from build123d import *

# Parameters (mm, degrees)
BOSS_EXTRUDE1_DEPTH = 3.175


with BuildPart() as part:
    # Sketch1 → Boss-Extrude1 (new body)
    with BuildSketch(Plane.XY):
        with BuildLine():
            Line((0, 0), (0, 3.175))
            Line((0, 3.175), (-3.175, 3.175))
            Line((-3.175, 3.175), (-3.175, 6.35))
            Line((-3.175, 6.35), (0, 6.35))
            Line((0, 6.35), (0, 7.62))
            Line((0, 7.62), (9.525, 7.62))
            Line((9.525, 7.62), (9.525, 5.582477749))
            Line((9.525, 5.582477749), (12.7, 5.582477749))
            Line((12.7, 5.582477749), (12.7, 7.62))
            Line((12.7, 7.62), (14.224, 7.62))
            Line((14.224, 7.62), (14.224, 11.43))
            Line((14.224, 11.43), (12.7, 11.43))
            Line((12.7, 11.43), (12.7, 13.467522251))
            Line((12.7, 13.467522251), (9.525, 13.467522251))
            Line((9.525, 13.467522251), (9.525, 11.43))
            Line((9.525, 11.43), (0, 11.43))
            Line((0, 11.43), (0, 12.7))
            Line((0, 12.7), (-3.175, 12.7))
            Line((-3.175, 12.7), (-3.175, 15.875))
            Line((-3.175, 15.875), (0, 15.875))
            Line((0, 15.875), (0, 19.05))
            Line((0, 19.05), (3.175, 19.05))
            Line((3.175, 19.05), (3.175, 22.225))
            Line((3.175, 22.225), (12.7, 22.225))
            Line((12.7, 22.225), (12.7, 19.05))
            Line((12.7, 19.05), (15.875, 19.05))
            ThreePointArc((15.875, 19.05), (29.345384182, 13.470384182), (34.925, 0))
            Line((34.925, 0), (25.4, 0))
            Line((25.4, 0), (25.4, -3.175))
            Line((25.4, -3.175), (15.875, -3.175))
            Line((15.875, -3.175), (15.875, 0))
            Line((15.875, 0), (0, 0))
        make_face()
    extrude(amount=BOSS_EXTRUDE1_DEPTH)


solid = part.part
For this review, take the finished solid that the model builds, in its own axes (mm). A direction names the side the tool comes from. Give positions to 0.01 mm unless a question says otherwise; leave off trailing zeros. Loops run counter-clockwise (first coordinate to the right, second up) from the corner with the lowest first, then second, coordinate; pieces in that order, holes last. Notation, with made-up numbers: (75.25, 84) - (131.25, 84) arc R16 cw to (131.25, 113) - close; hole circle Ø3 at (71.25, 63.5). An arc over 180 degrees is marked (long way). Write each question's results on one line, items separated by ' | '.
(1) Take a section at C-C (y = -1). Give the boundary of the cut face in (x, z) (3 decimals), then the cut area to 3 significant figures.
Conclusion:
outline: (15.875, 0) - (25.4, 0) - (25.4, 3.175) - (15.875, 3.175) - close | area: 30.2 mm^2
(2) Take a section at A-A (x = 2.5). Give the boundary of the cut face in (y, z) (3 decimals), then the cut area to 3 significant figures.
Conclusion:
outline: (0, 0) - (7.62, 0) - (7.62, 3.175) - (0, 3.175) - close; (11.43, 0) - (19.05, 0) - (19.05, 3.175) - (11.43, 3.175) - close | area: 48.4 mm^2
(3) For pin 1 Ø1.2 at (x, z) = (13.5, 2.5) entering from -Y; pin 2 Ø1.6 at (x, z) = (-1, 1) entering from -Y (3 decimals); pin 3 Ø1 at (y, z) = (-1, 2) entering from -X (3 decimals); pin 4 Ø0.6 at (y, z) = (12.5, 1.5) entering from -X (3 decimals), all flat-tipped, find the tip position at first contact; note any pin that passes through.
Conclusion:
pin 1: y = 0 | pin 2: y = 3.175 | pin 3: x = 15.875 | pin 4: x = -3.175
(4) Draft analysis for pull direction Y (two halves, no side actions). For faces 1 (the flat face through (-2, 15.875, 2)), 2 (the flat face through (15.875, -2, 2)), 3 (the flat face through (9.525, 7, 2)), state which applies: +Y half, -Y half, draft (parallel to the pull), parting line (faces both ways), or undercut.
Conclusion:
face 1: +Y half | face 2: draft | face 3: undercut
(5) For line 1 along Y through (x, z) = (12, 1) (3 decimals); line 2 along Y through (x, z) = (-1, 1.6) (3 decimals); line 3 along X through (y, z) = (19.5, 0.5) (3 decimals), list the stretches that pass through material, from the lowest coordinate up.
Conclusion:
line 1: 0 to 5.582, 13.468 to 22.225 | line 2: 3.175 to 6.35, 12.7 to 15.875 | line 3: 3.175 to 12.7
(6) Take a section at D-D (x = 22). Give the boundary of the cut face in (y, z) (3 decimals), then the cut area to 3 significant figures.
Conclusion:
outline: (-3.175, 0) - (18.038, 0) - (18.038, 3.175) - (-3.175, 3.175) - close | area: 67.4 mm^2
(7) For faces 4 (the flat face through (0, 17, 2)), 5 (the flat face through (9.525, 12, 2)), 6 (the flat face through (14, 19.05, 2)), list the 3-axis set-ups (+Z, -Z, +X, -X, +Y, -Y) from which the entire face can be reached by the end or side of a thin tool; tool diameter is ignored.
Conclusion:
face 4: +Z, -Z, -X, +Y | face 5: +Z, -Z | face 6: +Z, -Z, +X, +Y
